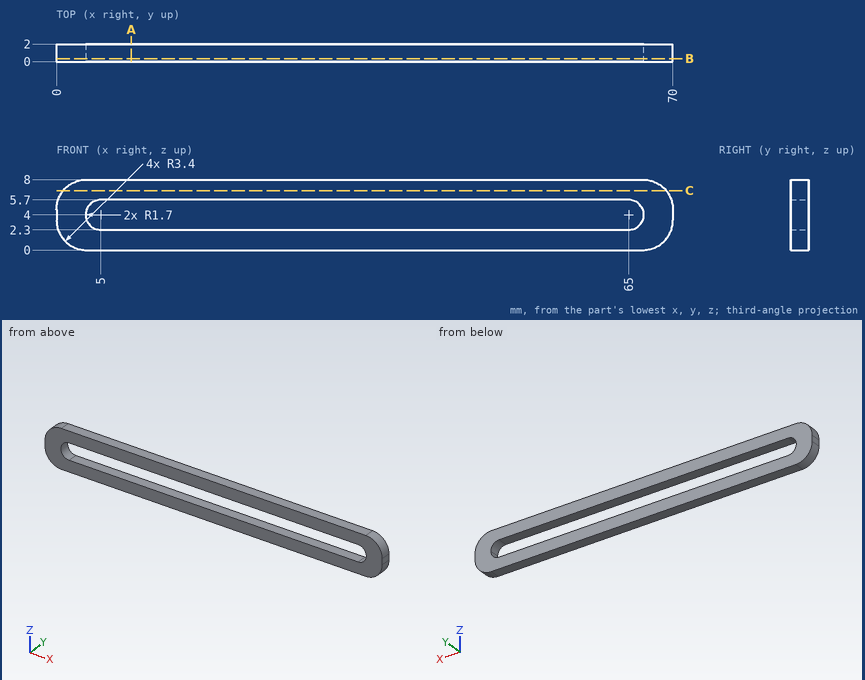
Print and shaded views of the part. All mm, measured from the part's lowest x, y and z. Give positions to 0.01 mm unless a question says otherwise; leave off trailing zeros. Loops run counter-clockwise (first coordinate to the right, second up) from the corner with the lowest first, then second, coordinate; pieces in that order, holes last. Notation, with made-up numbers: (30.25, 2) -> (72.25, 2) arc R13 cw to (72.25, 21) -> close; hole circle Ø5 at (1, 60.5). An arc over 180 degrees is marked (long way). Use CSV: the item, a comma, the result in double quotes. Start each with the question number.
1) Wall check: line 1 (Z direction, x = 37, y = 1.05); line 2 (Z direction, x = 66.5, y = 1.5); line 3 (X direction, y = 1.65, z = 4.75). Give the ranges that are in metal, low to high.
2) Slice it at B-B on y = 0.35. Give the cut face in (x, z), plus the area to 3 significant figures.
3) Flat gauge pin, fed straight in: pin 1 Ø0.6 at (x, y) = (36.5, 0.5) entering from -Z. Where does the tip first touch, or does it go through?
4) Slice it at C-C on z = 6.75. Give the cut face in (x, y), plus the area to 3 significant figures.
5) Slice it at A-A on x = 8.5. Give the cut face in (y, z).
Computed values:
1,line 1,"z = 0 to 2.3, 5.7 to 8"
1,line 2,"z = 0 to 3.2, 4.8 to 8"
1,line 3,"x = 0 to 3.47, 66.53 to 70"
2,outline,"(0, 3.4) arc R3.4 ccw to (3.4, 0) -> (66.6, 0) arc R3.4 ccw to (70, 3.4) -> (70, 4.6) arc R3.4 ccw to (66.6, 8) -> (3.4, 8) arc R3.4 ccw to (0, 4.6) -> close; hole (5, 2.3) -> (65, 2.3) arc R1.7 ccw to (65, 5.7) -> (5, 5.7) arc R1.7 ccw to start"
2,area,"337 mm^2"
3,pin 1,"stops at z = 0"
4,outline,"(0.77, 0) -> (69.23, 0) -> (69.23, 2) -> (0.77, 2) -> close"
4,area,"137 mm^2"
5,outline,"(0, 0) -> (2, 0) -> (2, 2.3) -> (0, 2.3) -> close; (0, 5.7) -> (2, 5.7) -> (2, 8) -> (0, 8) -> close"
